For this review, use the dimensioned drawing (mm, ordinates from the lowest corner) and the shaded views. Give positions to 0.01 mm unless a question says otherwise; leave off trailing zeros. Use a Markdown table: item, result. Add a question column.
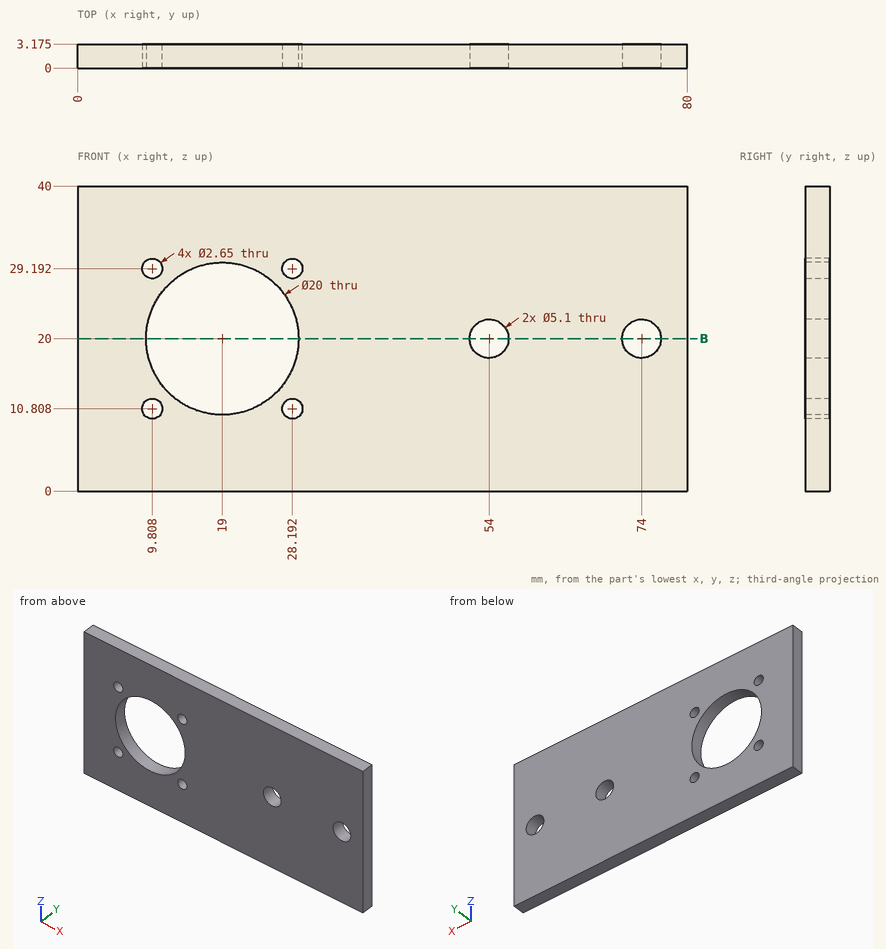
Q1. We need section B-B (z = 20). Count the separate pieces of the cut face and the enclosed holes in it, plus the area to 3 significant figures.
Q2. Clearance check with a flat-ended pin moving along its axis: P1, Ø3, axis at x = 54, z = 20, coming from the +Y side. State where the tip first meets the part, or that it passes through.
Q3. Wall thickness on probe 1 along X at (y, z) = (2.1, 20); probe 2 along X at (y, z) = (1.6, 28.5) (1 decimal); probe 3 along Z at (x, y) = (54, 0.9): over which ranges is each line inside the solid? List them lowest first.
Here are the results:
| question | item | result |
|---|---|---|
| 1 | separate pieces | 4 |
| 1 | enclosed holes | 0 |
| 1 | area | 158 mm2 |
| 2 | P1 | through |
| 3 | probe 1 | 0 to 9, 29 to 51.45, 56.55 to 71.45, 76.55 to 80 |
| 3 | probe 2 | 0 to 8.7, 10.9 to 13.7, 24.3 to 27.1, 29.3 to 80 |
| 3 | probe 3 | 0 to 17.45, 22.55 to 40 |
